Part model, mm, in its own coordinate system. Round coordinates to 2 decimals unless told otherwise and drop trailing zeros. Loops run counter-clockwise (first coordinate to the right, second up) from the corner with the lowest first, then second, coordinate; pieces in that order, holes last.
from build123d import *

# Parameters (mm, degrees)
F0_R     = 32.639
F0_R_2   = 29.591
F1_DEPTH = 5.08
F0_R_3   = 5.715
F2_DEPTH = 2.54


with BuildPart() as f1:
    # F0 (on Top) → F1 (new body)
    with BuildSketch(Plane.XY):
        Circle(F0_R)
        Circle(F0_R_2, mode=Mode.SUBTRACT)
    extrude(amount=F1_DEPTH)

    # F0 (on Top) → F2 (join)
    with BuildSketch(Plane.XY):
        Circle(F0_R_2)
        with Locations((-17.302921, -16.291201)):
            Circle(F0_R_3, mode=Mode.SUBTRACT)
        Circle(F0_R_3, mode=Mode.SUBTRACT)
    extrude(amount=F2_DEPTH)


solid = f1.part
1) Slice it at D-D, the plane z = 4.3. Give the cut face in (x, y).
Values:
outline: circle Ø65.28 at (0, 0); hole circle Ø59.18 at (0, 0)
2) Slice it at C-C, the plane y = -7. Give the cut face in (x, z).
Values:
outline: (-31.88, 0) - (31.88, 0) - (31.88, 5.08) - (28.75, 5.08) - (28.75, 2.54) - (-28.75, 2.54) - (-28.75, 5.08) - (-31.88, 5.08) - close
3) Mould opens along X. For faces 1 (the face through (7, -29, 5.08)), 2 (the face through (6, 0, 2.54)), 3 (the face through (-6.41, -28.89, 3.79)), 4 (the face through (30.15, -12.5, 2.5)) say: released by +X, released by -X, zero draft, split by the parting line, or undercut.
Values:
face 1: zero draft
face 2: undercut
face 3: undercut
face 4: split by the parting line
4) Drop flat-ended pins along their axis: pin 1 Ø6 at (x, y) = (-21.5, -14.5) entering from -Z; pin 2 Ø1.5 at (x, z) = (14, 2) entering from +Y; pin 3 Ø3 at (x, z) = (13, 2) entering from +Y; pin 4 Ø3 at (x, y) = (25.5, -6.5) entering from +Z. Give the stop position or say it passes through.
Values:
pin 1: stops at z = 0
pin 2: stops at y = 29.83
pin 3: stops at y = 30.55
pin 4: stops at z = 2.54
5) Slice it at A-A, the plane y = 0. Give the cut face in (x, z) (3 decimals), then the cut area to 3 significant figures.
Values:
outline: (-32.639, 0) - (-5.715, 0) - (-5.715, 2.54) - (-29.591, 2.54) - (-29.591, 5.08) - (-32.639, 5.08) - close; (5.715, 0) - (32.639, 0) - (32.639, 5.08) - (29.591, 5.08) - (29.591, 2.54) - (5.715, 2.54) - close
area: 152 mm2
6) Wall check: line 1 along Y through (x, z) = (0, 0.85) (3 decimals); line 2 along Y through (x, z) = (0, 4.2); line 3 along Z through (x, y) = (-5, 22). Give the ranges that are in metal, low to high.
Values:
line 1: y = -32.639 to -5.715, 5.715 to 32.639
line 2: y = -32.64 to -29.59, 29.59 to 32.64
line 3: z = 0 to 2.54
7) Slice it at B-B, the plane x = -2.5. Give the cut face in (y, z), then the cut area to 3 significant figures.
Values:
outline: (-32.54, 0) - (-5.14, 0) - (-5.14, 2.54) - (-29.49, 2.54) - (-29.49, 5.08) - (-32.54, 5.08) - close; (5.14, 0) - (32.54, 0) - (32.54, 5.08) - (29.49, 5.08) - (29.49, 2.54) - (5.14, 2.54) - close
area: 155 mm2
